from build123d import *

# Parameters (mm, degrees)
F0_W          = 6.35
F0_H          = 12.7
F1_DEPTH      = 12.7
F3_DEPTH      = 6.351
F3_DEPTH_BACK = 6.351
F5_DEPTH      = 6.351
F5_DEPTH_BACK = 6.351
F7_DEPTH      = 6.351
F7_DEPTH_BACK = 6.351


# Not quite as in the source:
# - a pattern or mirror of a feature is missing from the dataset's text; its kind, count and spacing are read off the source's solid


with BuildPart() as f1:
    # F0 (on Right) → F1 (new body, symmetric)
    with BuildSketch(Plane.YZ):
        Rectangle(F0_W, F0_H)
    extrude(amount=F1_DEPTH, both=True)

    # F2 (on Top) → F3 (cut, two sides)
    with BuildSketch(Plane.XY) as f3_sk:
        Polygon((-12.7, 3.175), (-12.7, 0), (-5.0348719395, 3.175), align=None)
    f3 = extrude(amount=-F3_DEPTH, mode=Mode.SUBTRACT) + extrude(f3_sk.sketch, amount=F3_DEPTH_BACK, mode=Mode.SUBTRACT)

    # F3_copies: F3 across plane
    add(f3.mirror(Plane(origin=(0, 0, 0), x_dir=(0, 0, -1), z_dir=(0, -1, 0))), mode=Mode.SUBTRACT)

    # F4 (on Top) → F5 (cut, two sides)
    with BuildSketch(Plane.XY) as f5_sk:
        Polygon((17.9670583457, 3.175), (7.5919586605, 3.175), (12.7, 1.05918), align=None)
    extrude(amount=-F5_DEPTH, mode=Mode.SUBTRACT)
    extrude(f5_sk.sketch, amount=F5_DEPTH_BACK, mode=Mode.SUBTRACT)

    # F6 (on Top) → F7 (cut, two sides)
    with BuildSketch(Plane.XY) as f7_sk:
        Polygon((12.7, 1.05918), (10.9461452185, -3.175), (12.7, -3.175), align=None)
    extrude(amount=-F7_DEPTH, mode=Mode.SUBTRACT)
    extrude(f7_sk.sketch, amount=F7_DEPTH_BACK, mode=Mode.SUBTRACT)


solid = f1.part
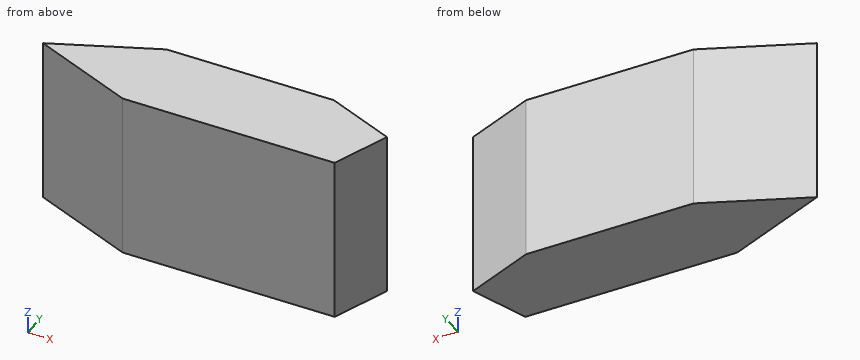
Can you work these out from the model? Positions are in its coordinate system, mm. Coordinates: 2 decimals unless noted, no trailing zeros. Write each loop counter-clockwise with the first axis right and the second up, starting at its lowest first coordinate (ties: lowest second). Pieces come first, ordered by that corner, then holes. Notation, with made-up numbers: (62, -11) -> (74, -11) arc R26 ccw to (74, 25) -> close; hole circle Ø7 at (6, 64.5). An arc over 180 degrees is marked (long way). Write each question's results on one line, items separated by ' | '. Start each with the question number.
Q1. I'm going to push a flat-ended pin straight in: pin 1 (1 mm diameter, centred on y = -1, z = -1, fed in from +X). Where does the tip first touch, or does it pass through?
Q2. Imagine slicing it at B-B (y = 0.25). Write out the boundary of the cut face in (x, z).
Q3. If I drill on probe 1 along Y at (x, z) = (-6.5, 4.5); probe 2 along X at (y, z) = (2.25, 4.25); probe 3 along Y at (x, z) = (-6, 0), over which ranges is the centre line in solid material (lowest first)?
Q4. Imagine slicing it at A-A (z = -3.5). Write out the boundary of the cut face in (x, y) (3 decimals).
Q5. Imagine slicing it at C-C (x = -8). Write out the boundary of the cut face in (y, z).
Taken from the geometry:
1) pin 1: stops at x = 12.05
2) outline: (-12.1, -6.35) -> (12.36, -6.35) -> (12.36, 6.35) -> (-12.1, 6.35) -> close
3) probe 1: y = -2.57 to 2.57 | probe 2: x = -7.27 to 9.83 | probe 3: y = -2.78 to 2.78
4) outline: (-12.7, 0) -> (-5.035, -3.175) -> (10.946, -3.175) -> (12.7, 1.059) -> (7.592, 3.175) -> (-5.035, 3.175) -> close
5) outline: (-1.95, -6.35) -> (1.95, -6.35) -> (1.95, 6.35) -> (-1.95, 6.35) -> close
